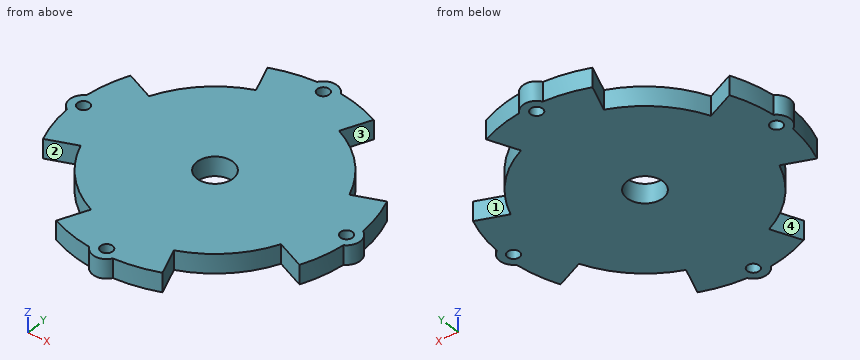
from build123d import *

# Parameters (mm, degrees)
SKETCH1_R           = 1.25
SKETCH1_R_2         = 3.75
BOSS_EXTRUDE2_DEPTH = 4


with BuildPart() as part:
    # Sketch1 → Boss-Extrude2 (new body)
    with BuildSketch(Plane.XY):
        with BuildLine():
            Line((-21.249229248, 8.801718944), (-27.195761321, 11.264853178))
            ThreePointArc((-27.195761321, 11.264853178), (-28.600693627, 6.964673358), (-29.330127019, 2.5))
            ThreePointArc((-29.330127019, 2.5), (-30.773502692, 0), (-29.330127019, -2.5))
            ThreePointArc((-29.330127019, -2.5), (-28.600693627, -6.964673358), (-27.195761321, -11.264853178))
            Line((-27.195761321, -11.264853178), (-21.249229248, -8.801718944))
            ThreePointArc((-21.249229248, -8.801718944), (-16.263455967, -16.263455967), (-8.801718944, -21.249229248))
            Line((-8.801718944, -21.249229248), (-11.264853178, -27.195761321))
            ThreePointArc((-11.264853178, -27.195761321), (-6.964673358, -28.600693627), (-2.5, -29.330127019))
            ThreePointArc((-2.5, -29.330127019), (0, -30.773502692), (2.5, -29.330127019))
            ThreePointArc((2.5, -29.330127019), (6.964673358, -28.600693627), (11.264853178, -27.195761321))
            Line((11.264853178, -27.195761321), (8.801718944, -21.249229248))
            ThreePointArc((8.801718944, -21.249229248), (16.263455967, -16.263455967), (21.249229248, -8.801718944))
            Line((21.249229248, -8.801718944), (27.195761321, -11.264853178))
            ThreePointArc((27.195761321, -11.264853178), (28.600693627, -6.964673358), (29.330127019, -2.5))
            ThreePointArc((29.330127019, -2.5), (30.773502692, 0), (29.330127019, 2.5))
            ThreePointArc((29.330127019, 2.5), (28.600693627, 6.964673358), (27.195761321, 11.264853178))
            Line((27.195761321, 11.264853178), (21.249229248, 8.801718944))
            ThreePointArc((21.249229248, 8.801718944), (16.263455967, 16.263455967), (8.801718944, 21.249229248))
            Line((8.801718944, 21.249229248), (11.264853178, 27.195761321))
            ThreePointArc((11.264853178, 27.195761321), (6.964673358, 28.600693627), (2.5, 29.330127019))
            ThreePointArc((2.5, 29.330127019), (0, 30.773502692), (-2.5, 29.330127019))
            ThreePointArc((-2.5, 29.330127019), (-6.964673358, 28.600693627), (-11.264853178, 27.195761321))
            Line((-11.264853178, 27.195761321), (-8.801718944, 21.249229248))
            ThreePointArc((-8.801718944, 21.249229248), (-16.263455967, 16.263455967), (-21.249229248, 8.801718944))
        make_face()
        with Locations((0, -27.886751346)):
            Circle(SKETCH1_R, mode=Mode.SUBTRACT)
        Circle(SKETCH1_R_2, mode=Mode.SUBTRACT)
        with Locations((27.886751346, 0)):
            Circle(SKETCH1_R, mode=Mode.SUBTRACT)
        with Locations((-27.886751346, 0)):
            Circle(SKETCH1_R, mode=Mode.SUBTRACT)
        with Locations((0, 27.886751346)):
            Circle(SKETCH1_R, mode=Mode.SUBTRACT)
    extrude(amount=BOSS_EXTRUDE2_DEPTH)


solid = part.part
The listing builds one solid part. Answer for the finished solid, in the listing's coordinates (mm). Face numbers are marked on the shaded views. A direction names the side the tool comes from. Give positions to 0.01 mm unless a question says otherwise; leave off trailing zeros. Order: outer loops, then holes, each group sorted by start corner. A loop starts at its lowest first (then second) coordinate and runs counter-clockwise, first axis right, second up. Notation, with made-up numbers: (77, 58) - (112, 58) arc R14 cw to (112, 84) - close; hole circle Ø4 at (-14, 61). An arc over 180 degrees is marked (long way). One line per item, written item: value. Start each with the question number.
1) Find the intervals of material crossed by L1, parallel to Y at x = -11, z = 3.8; L2, parallel to X at y = -1.5, z = 0.65; L3, parallel to X at y = -2, z = 1.2, in increasing order.
2) A cutting plane is placed at A-A on x = 0. Give the vertices of the cut face in (y, z), then the cut area to 3 significant figures.
3) Given pin 1 Ø1.5 at (y, z) = (-4.5, 3.5) entering from -X; pin 2 Ø1 at (x, z) = (-21.5, 2.5) entering from +Y, each flat-ended and moving along its own axis, determine where each tip first touches the part or whether it passes through.
4) A tool of negligible diameter and unlimited length cuts with its end or side. For the marked faces 1, 2, 3 and 4, from which of +Z, -Z, +X, -X, +Y, -Y can it reach the whole face along a straight path? Write none if from no direction.
5) A cutting plane is placed at C-C on z = 2.7. State how many separate pieces and enclosed holes the cut face has, then the cut area to 3 significant figures.
6) A cutting plane is placed at D-D on x = -17.5. Give the vertices of the cut face in (y, z).
Answer sheet:
1. L1: y = -27.3 to -26.56, -20.2 to 20.2, 26.56 to 27.3
1. L2: x = -30.35 to -3.44, 3.44 to 30.35
1. L3: x = -29.97 to -3.17, 3.17 to 29.97
2. outline: (-30.77, 0) - (-29.14, 0) - (-29.14, 4) - (-30.77, 4) - close; (-26.64, 0) - (-3.75, 0) - (-3.75, 4) - (-26.64, 4) - close; (3.75, 0) - (26.64, 0) - (26.64, 4) - (3.75, 4) - close; (29.14, 0) - (30.77, 0) - (30.77, 4) - (29.14, 4) - close
2. area: 196 mm2
3. pin 1: stops at x = -29.2
3. pin 2: stops at y = 9.38
4. face 1: +Z, -Z, +Y
4. face 2: +Z, -Z, -Y
4. face 3: +Z, -Z, +X
4. face 4: +Z, -Z, -X
5. separate pieces: 1
5. enclosed holes: 5
5. area: 2,150 mm2
6. outline: (-14.92, 0) - (14.92, 0) - (14.92, 4) - (-14.92, 4) - close
